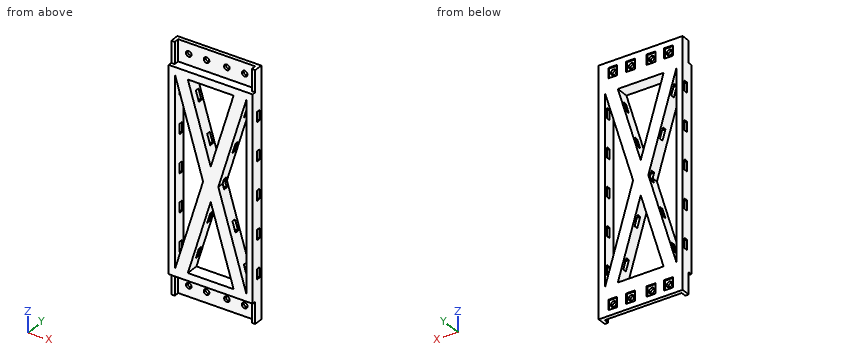
```python
from build123d import *

# Parameters (mm, degrees)
SKETCH1_W           = 66
SKETCH1_H           = 193.8
BOSS_EXTRUDE1_DEPTH = 10
SKETCH2_W           = 66
SKETCH2_H           = 17
CUT_EXTRUDE1_DEPTH  = 3
SKETCH3_W           = 66
SKETCH3_H           = 17
CUT_EXTRUDE2_DEPTH  = 3
SKETCH4_W           = 60.6
SKETCH4_H           = 4
CUT_EXTRUDE3_DEPTH  = 17
SKETCH5_W           = 60.6
SKETCH5_H           = 4
CUT_EXTRUDE4_DEPTH  = 17
SKETCH6_R           = 2.2
CUT_EXTRUDE5_DEPTH  = 10
SKETCH7_W           = 7
SKETCH7_H           = 8
CUT_EXTRUDE6_DEPTH  = 1
CUT_EXTRUDE7_DEPTH  = 271.07407236
SKETCH9_W           = 8
SKETCH9_H           = 3
CUT_EXTRUDE8_DEPTH  = 127.422870419


with BuildPart() as part:
    # Sketch1 → Boss-Extrude1 (new body)
    with BuildSketch(Plane(origin=(0, 0, 0), x_dir=(1, 0, 0), z_dir=(0, 1, 0))):
        with Locations((214.615149771, -10.462666532)):
            Rectangle(SKETCH1_W, SKETCH1_H)
    extrude(amount=BOSS_EXTRUDE1_DEPTH)

    # Sketch2 → Cut-Extrude1 (cut)
    with BuildSketch(Plane.XZ):
        with Locations((214.615149771, -77.937333468)):
            Rectangle(SKETCH2_W, SKETCH2_H)
    extrude(amount=-CUT_EXTRUDE1_DEPTH, mode=Mode.SUBTRACT)

    # Sketch3 → Cut-Extrude2 (cut)
    with BuildSketch(Plane.XZ):
        with Locations((214.615149771, 98.862666532)):
            Rectangle(SKETCH3_W, SKETCH3_H)
    extrude(amount=-CUT_EXTRUDE2_DEPTH, mode=Mode.SUBTRACT)

    # Sketch4 → Cut-Extrude3 (cut)
    with BuildSketch(Plane(origin=(0, 0, -86.437333468), x_dir=(-1, 0, 0), z_dir=(0, 0, -1))):
        with Locations((-214.615149771, 5)):
            Rectangle(SKETCH4_W, SKETCH4_H)
    extrude(amount=-CUT_EXTRUDE3_DEPTH, mode=Mode.SUBTRACT)

    # Sketch5 → Cut-Extrude4 (cut)
    with BuildSketch(Plane.XY.offset(107.362666532)):
        with Locations((214.615149771, 5)):
            Rectangle(SKETCH5_W, SKETCH5_H)
    extrude(amount=-CUT_EXTRUDE4_DEPTH, mode=Mode.SUBTRACT)

    # Sketch6 → Cut-Extrude5 (cut)
    with BuildSketch(Plane.XZ):
        with Locations(Location((236.615149771, 98.962666532, 0), (0, 0, 90))):
            Circle(SKETCH6_R)
        with Locations(Location((222.615149771, 98.962666532, 0), (0, 0, 90))):
            Circle(SKETCH6_R)
        with Locations(Location((206.615149771, 98.962666532, 0), (0, 0, 90))):
            Circle(SKETCH6_R)
        with Locations(Location((192.615149771, 98.962666532, 0), (0, 0, 90))):
            Circle(SKETCH6_R)
        with Locations(Location((236.615149771, -78.037333468, 0), (0, 0, 90))):
            Circle(SKETCH6_R)
        with Locations(Location((222.615149771, -78.037333468, 0), (0, 0, 90))):
            Circle(SKETCH6_R)
        with Locations(Location((206.615149771, -78.037333468, 0), (0, 0, 90))):
            Circle(SKETCH6_R)
        with Locations(Location((192.615149771, -78.037333468, 0), (0, 0, 90))):
            Circle(SKETCH6_R)
    extrude(amount=-CUT_EXTRUDE5_DEPTH, mode=Mode.SUBTRACT)

    # Sketch7 → Cut-Extrude6 (cut)
    with BuildSketch(Plane(origin=(0, 10, 0), x_dir=(1, 0, 0), z_dir=(0, 1, 0))):
        with Locations((192.615149771, 78.037333468)):
            Rectangle(SKETCH7_W, SKETCH7_H)
        with Locations((206.615149771, 78.037333468)):
            Rectangle(SKETCH7_W, SKETCH7_H)
        with Locations((222.615149771, 78.037333468)):
            Rectangle(SKETCH7_W, SKETCH7_H)
        with Locations((236.615149771, 78.037333468)):
            Rectangle(SKETCH7_W, SKETCH7_H)
        with Locations((236.615149771, -98.962666532)):
            Rectangle(SKETCH7_W, SKETCH7_H)
        with Locations((222.615149771, -98.962666532)):
            Rectangle(SKETCH7_W, SKETCH7_H)
        with Locations((206.615149771, -98.962666532)):
            Rectangle(SKETCH7_W, SKETCH7_H)
        with Locations((192.615149771, -98.962666532)):
            Rectangle(SKETCH7_W, SKETCH7_H)
    extrude(amount=-CUT_EXTRUDE6_DEPTH, mode=Mode.SUBTRACT)

    # Sketch8 → Cut-Extrude7 (cut, through all)
    with BuildSketch(Plane(origin=(0, 10, 0), x_dir=(1, 0, 0), z_dir=(0, 1, 0))):
        Polygon((186.615149771, 63.437333468), (186.615149771, -84.362666532), (208.615149771, -10.462666532), align=None)
        Polygon((196.615149771, 63.437333468), (214.615149771, 2.973697104), (232.615149771, 63.437333468), align=None)
        Polygon((214.615149771, -23.899030169), (196.615149771, -84.362666532), (232.615149771, -84.362666532), align=None)
        Polygon((242.615149771, 63.437333468), (242.615149771, -84.362666532), (220.615149771, -10.462666532), align=None)
    extrude(amount=-CUT_EXTRUDE7_DEPTH, mode=Mode.SUBTRACT)

    # Sketch9 → Cut-Extrude8 (cut, through all)
    with BuildSketch(Plane(origin=(247.615149771, 0, 0), x_dir=(0, 0, -1), z_dir=(1, 0, 0))):
        with Locations((-70.462666532, 6.5)):
            Rectangle(SKETCH9_W, SKETCH9_H)
        with Locations((-40.462666532, 6.5)):
            Rectangle(SKETCH9_W, SKETCH9_H)
        with Locations((-10.462666532, 6.5)):
            Rectangle(SKETCH9_W, SKETCH9_H)
        with Locations((19.537333468, 6.5)):
            Rectangle(SKETCH9_W, SKETCH9_H)
        with Locations((49.537333468, 6.5)):
            Rectangle(SKETCH9_W, SKETCH9_H)
    extrude(amount=-CUT_EXTRUDE8_DEPTH, mode=Mode.SUBTRACT)


solid = part.part
```
Source: CAD feature listing. Evaluate the final solid. Frame: model axes, mm. Coordinates: 2 decimals unless noted, no trailing zeros. Write each loop counter-clockwise with the first axis right and the second up, starting at its lowest first coordinate (ties: lowest second). Pieces come first, ordered by that corner, then holes. Notation, with made-up numbers: (62.5, 4) - (66.5, 4) arc R25 ccw to (66.5, 39) - close; hole circle Ø8 at (16, 21). An arc over 180 degrees is marked (long way). Answer as a JSON object with one key per item and string values.
Q1. Section query A-A, the plane z = -31. Output: boundary loops of the cut face in (x, y).
Ans:
{"outline": "(181.62, 0) - (186.62, 0) - (186.62, 10) - (181.62, 10) - close; (196.27, 0) - (206.27, 0) - (206.27, 10) - (196.27, 10) - close; (222.96, 0) - (232.96, 0) - (232.96, 10) - (222.96, 10) - close; (242.62, 0) - (247.62, 0) - (247.62, 10) - (242.62, 10) - close"}
Q2. Section query B-B, the plane y = 1.5. Output: boundary loops of the cut face in (x, z), plus the area to 3 significant figures.
Ans:
{"outline": "(181.62, -69.44) - (247.62, -69.44) - (247.62, 90.36) - (181.62, 90.36) - close; hole (186.62, -63.44) - (208.62, 10.46) - (186.62, 84.36) - close; hole (196.62, -63.44) - (232.62, -63.44) - (214.62, -2.97) - close; hole (196.62, 84.36) - (214.62, 23.9) - (232.62, 84.36) - close; hole (220.62, 10.46) - (242.62, -63.44) - (242.62, 84.36) - close", "area": "5,120 mm2"}
Q3. Material intervals for line 1 (X direction, y = 7.5, z = 30.5); line 2 (X direction, y = 2, z = 83.5); line 3 (Y direction, x = 225.5, z = 40.5), sorted ascending. Write a range as [from, to].
Ans:
{"line 1": "x = [181.62, 186.62], [202.65, 212.65], [216.58, 226.58], [242.62, 247.62]", "line 2": "x = [181.62, 186.62], [186.87, 196.87], [232.36, 242.36], [242.62, 247.62]", "line 3": "y = [0, 5], [8, 10]"}
Q4. First-contact query: pin 1 Ø0.9 at (x, y) = (185, 6) entering from +Z. Flat tip, straight axial feed; report the tip coordinate or a pass-through.
Ans:
{"pin 1": "stops at z = 90.36"}
